Geometry check sheet. Reference: the model listing, model coordinates, mm. A direction names the side the tool comes from. Round coordinates to 2 decimals unless told otherwise and drop trailing zeros. Order: outer loops, then holes, each group sorted by start corner. A loop starts at its lowest first (then second) coordinate and runs counter-clockwise, first axis right, second up. Notation, with made-up numbers: M 78.5,-18 L 135.5,-18 A12 cw 135.5,4 Z; hole C -18.5,61 d5. An arc over 180 degrees is marked long. Return JSON: item names as keys, results as strings. Group by question number.
```python
from build123d import *

# Parameters (mm, degrees)
CUT_EXTRUDE1_DEPTH  = 12
SKETCH6_R           = 4.25
BOSS_EXTRUDE1_DEPTH = 5
SKETCH7_R           = 2.067
CUT_EXTRUDE2_DEPTH  = 40.361021372
SKETCH8_R           = 2.5
BOSS_EXTRUDE2_DEPTH = 18
CUT_EXTRUDE3_DEPTH  = 2
TAP1_D              = 4.134
TAP1_DEPTH          = 5.3


with BuildPart() as part:
    # Sketch1 → Revolve1 (revolve)
    with BuildSketch(Plane.XY, mode=Mode.PRIVATE) as revolve1_sk:
        Polygon((-26.6, -14), (-9.3, -14), (-9.3, -15.25), (-21.3, -15.75), (-21.3, -23), (-23.1, -23), (-23.1, -25), (-26.6, -25), align=None)
    revolve(revolve1_sk.sketch.rotate(Axis((0, 0, 0), (-1, 0, 0)), 180), axis=Axis((0, 0, 0), (-1, 0, 0)))

    # Sketch2 → Cut-Extrude1 (cut)
    with BuildSketch(Plane(origin=(-9.3, 0, 0), x_dir=(0, 0, -1), z_dir=(1, 0, 0))):
        with BuildLine():
            Line((0.5, -13.99106858), (0.5, -15.742061491))
            ThreePointArc((0.5, -15.742061491), (0, -15.75), (-0.5, -15.742061491))
            Line((-0.5, -15.742061491), (-0.5, -13.99106858))
            ThreePointArc((-0.5, -13.99106858), (0, -14), (0.5, -13.99106858))
        make_face()
    extrude(amount=-CUT_EXTRUDE1_DEPTH, mode=Mode.SUBTRACT)

    # Sketch3 → Revolve2 (revolve)
    with BuildSketch(Plane.XY, mode=Mode.PRIVATE) as revolve2_sk:
        Polygon((-17.3, -15.583333333), (0, -14.8625), (0, -23), (-17.3, -23), align=None)
    revolve(revolve2_sk.sketch.rotate(Axis((0, 0, 0), (-1, 0, 0)), 358.161317169), axis=Axis((0, 0, 0), (-1, 0, 0)))

    # Sketch4 for Cut-Loft1 → Cut-Loft1 section 0
    with BuildSketch(Plane(origin=(0, 0, 0), x_dir=(0, 0, -1), z_dir=(1, 0, 0))):
        with BuildLine():
            Line((6.531671834, 22.05305564), (4.288541607, 14.230330886))
            # circular arc as an exact rational Bezier (weights 1, cos(half-angle), 1)
            Bezier((4.288541607, 14.230330886), (4.097031168, 14.288045671), (3.904036928, 14.340585829), weights=[1, 0.999909455, 1])
            Line((3.904036928, 14.340585829), (6.147167155, 22.163310582))
            Bezier((6.147167155, 22.163310582), (6.339898882, 22.109854934), (6.531671834, 22.05305564), weights=[1, 0.999962192, 1])
        make_face()
    # Sketch5 for Cut-Loft1 → Cut-Loft1 section 1
    with BuildSketch(Plane.ZY.offset(17.3)):
        with BuildLine():
            Line((-6.531671834, 22.05305564), (-4.48724736, 14.923300202))
            Bezier((-4.48724736, 14.923300202), (-4.295702598, 14.980895286), (-4.102742682, 15.033555144), weights=[1, 0.999917638, 1])
            Line((-4.102742682, 15.033555144), (-6.147167155, 22.163310582))
            Bezier((-6.147167155, 22.163310582), (-6.339898882, 22.109854934), (-6.531671834, 22.05305564), weights=[1, 0.999962192, 1])
        make_face()
    loft(mode=Mode.SUBTRACT)

    # Sketch6 → Boss-Extrude1 (add)
    with BuildSketch(Plane.ZY.offset(26.6)):
        with Locations(Location((0, 19.4, 0), (0, 0, 90))):
            Circle(SKETCH6_R)
        with Locations(Location((10.280433726, -16.452133065, 0), (0, 0, 90))):
            Circle(SKETCH6_R)
        with Locations(Location((0, -19.4, 0), (0, 0, 90))):
            Circle(SKETCH6_R)
        with Locations(Location((-10.280433726, 16.452133065, 0), (0, 0, 90))):
            Circle(SKETCH6_R)
        with Locations(Location((10.280433726, 16.452133065, 0), (0, 0, 90))):
            Circle(SKETCH6_R)
        with Locations(Location((-10.280433726, -16.452133065, 0), (0, 0, 90))):
            Circle(SKETCH6_R)
        with Locations(Location((-18.648476901, 5.347364703, 0), (0, 0, 90))):
            Circle(SKETCH6_R)
        with Locations(Location((18.648476901, -5.347364703, 0), (0, 0, 90))):
            Circle(SKETCH6_R)
        with Locations(Location((18.648476901, 5.347364703, 0), (0, 0, 90))):
            Circle(SKETCH6_R)
        with Locations(Location((-18.648476901, -5.347364703, 0), (0, 0, 90))):
            Circle(SKETCH6_R)
    extrude(amount=BOSS_EXTRUDE1_DEPTH)

    # Sketch7 → Cut-Extrude2 (cut, through all)
    with BuildSketch(Plane.ZY.offset(17.3)):
        with Locations(Location((0, 19.4, 0), (0, 0, 270))):
            Circle(SKETCH7_R)
        with Locations(Location((10.280433726, -16.452133065, 0), (0, 0, 270))):
            Circle(SKETCH7_R)
        with Locations(Location((0, -19.4, 0), (0, 0, 270))):
            Circle(SKETCH7_R)
        with Locations(Location((-10.280433726, 16.452133065, 0), (0, 0, 270))):
            Circle(SKETCH7_R)
        with Locations(Location((10.280433726, 16.452133065, 0), (0, 0, 270))):
            Circle(SKETCH7_R)
        with Locations(Location((-10.280433726, -16.452133065, 0), (0, 0, 270))):
            Circle(SKETCH7_R)
        with Locations(Location((-18.648476901, 5.347364703, 0), (0, 0, 270))):
            Circle(SKETCH7_R)
        with Locations(Location((18.648476901, -5.347364703, 0), (0, 0, 270))):
            Circle(SKETCH7_R)
        with Locations(Location((18.648476901, 5.347364703, 0), (0, 0, 270))):
            Circle(SKETCH7_R)
        with Locations(Location((-18.648476901, -5.347364703, 0), (0, 0, 270))):
            Circle(SKETCH7_R)
    extrude(amount=-CUT_EXTRUDE2_DEPTH, mode=Mode.SUBTRACT)

    # Sketch8 → Boss-Extrude2 (add)
    with BuildSketch(Plane.ZY.offset(26.6)):
        with Locations(Location((0, 19.4, 0), (0, 0, 270))):
            Circle(SKETCH8_R)
        with Locations(Location((10.280433726, -16.452133065, 0), (0, 0, 270))):
            Circle(SKETCH8_R)
        with Locations(Location((0, -19.4, 0), (0, 0, 270))):
            Circle(SKETCH8_R)
        with Locations(Location((-10.280433726, 16.452133065, 0), (0, 0, 270))):
            Circle(SKETCH8_R)
        with Locations(Location((10.280433726, 16.452133065, 0), (0, 0, 270))):
            Circle(SKETCH8_R)
        with Locations(Location((-10.280433726, -16.452133065, 0), (0, 0, 270))):
            Circle(SKETCH8_R)
        with Locations(Location((-18.648476901, 5.347364703, 0), (0, 0, 270))):
            Circle(SKETCH8_R)
        with Locations(Location((18.648476901, -5.347364703, 0), (0, 0, 270))):
            Circle(SKETCH8_R)
        with Locations(Location((18.648476901, 5.347364703, 0), (0, 0, 270))):
            Circle(SKETCH8_R)
        with Locations(Location((-18.648476901, -5.347364703, 0), (0, 0, 270))):
            Circle(SKETCH8_R)
    extrude(amount=-BOSS_EXTRUDE2_DEPTH)

    # Sketch9 → Cut-Extrude3 (cut)
    with BuildSketch(Plane.ZY.offset(31.6)):
        Polygon((0, 21.709401077), (-2, 20.554700538), (-2, 18.245299462), (0, 17.090598923), (2, 18.245299462), (2, 20.554700538), align=None)
        Polygon((10.280433726, -14.142731989), (8.280433726, -15.297432527), (8.280433726, -17.606833604), (10.280433726, -18.761534142), (12.280433726, -17.606833604), (12.280433726, -15.297432527), align=None)
        Polygon((0, -17.090598923), (-2, -18.245299462), (-2, -20.554700538), (0, -21.709401077), (2, -20.554700538), (2, -18.245299462), align=None)
        Polygon((-10.280433726, 18.761534142), (-12.280433726, 17.606833604), (-12.280433726, 15.297432527), (-10.280433726, 14.142731989), (-8.280433726, 15.297432527), (-8.280433726, 17.606833604), align=None)
        Polygon((10.280433726, 18.761534142), (8.280433726, 17.606833604), (8.280433726, 15.297432527), (10.280433726, 14.142731989), (12.280433726, 15.297432527), (12.280433726, 17.606833604), align=None)
        Polygon((-10.280433726, -14.142731989), (-12.280433726, -15.297432527), (-12.280433726, -17.606833604), (-10.280433726, -18.761534142), (-8.280433726, -17.606833604), (-8.280433726, -15.297432527), align=None)
        Polygon((-18.648476901, 7.65676578), (-20.648476901, 6.502065241), (-20.648476901, 4.192664164), (-18.648476901, 3.037963626), (-16.648476901, 4.192664164), (-16.648476901, 6.502065241), align=None)
        Polygon((18.648476901, -3.037963626), (16.648476901, -4.192664164), (16.648476901, -6.502065241), (18.648476901, -7.65676578), (20.648476901, -6.502065241), (20.648476901, -4.192664164), align=None)
        Polygon((18.648476901, 7.65676578), (16.648476901, 6.502065241), (16.648476901, 4.192664164), (18.648476901, 3.037963626), (20.648476901, 4.192664164), (20.648476901, 6.502065241), align=None)
        Polygon((-18.648476901, -3.037963626), (-20.648476901, -4.192664164), (-20.648476901, -6.502065241), (-18.648476901, -7.65676578), (-16.648476901, -6.502065241), (-16.648476901, -4.192664164), align=None)
    extrude(amount=-CUT_EXTRUDE3_DEPTH, mode=Mode.SUBTRACT)

    # Tap1
    with Locations(Plane.ZY.offset(26.6)):
        with Locations((15.493528895, 11.675211449), (-15.493528895, -11.675211449), (-15.493528895, 11.675211449), (15.493528895, -11.675211449)):
            Hole(TAP1_D / 2, depth=TAP1_DEPTH)


solid = part.part
```
Q1. Set-up check for faces 4 (the face through (-29.065, -5.901, -22.862)), 5 (the face through (-15, -15, 0.5)), 6 (the face through (-8.6, -16, -10)): record each of +Z, -Z, +X, -X, +Y, -Y from which the full face is reachable in a straight line by a thin tool's end or side.
Q2. Depth check by flat-ended pin: pin 1 Ø1.5 at (x, z) = (-23.5, 2.5) entering from -Y; pin 2 Ø2 at (y, z) = (-20, -0.5) entering from +X; pin 3 Ø2 at (x, y) = (-30.5, 5.5) entering from +Z. Enter the tip coordinate at first touch or a pass-through.
Q3. Section check B-B on y = 0. Record the cut outline in (x, z).
Q4. Release check for a two-part mould opening along X. For faces 1 (the face through (-30.61, -18.19, 11.27)), 2 (the face through (-19.328, 18.436, 8.759)), 3 (the face through (0, -1, 16)) record: +X half, -X half, draft (parallel to the pull), parting line (faces both ways), or undercut.
Q5. Material ranges on line 1 along Z through (x, y) = (-4.75, -19.4); line 2 along X through (y, z) = (13, -12); line 3 along Z through (x, y) = (-26.5, 3), recorded low to high.
Q6. Section check A-A on x = -27.5. Count the separate pieces of the cut face and the enclosed holes in it, plus the area to 3 significant figures.
Geometry check:
{
 "1": {"face 4": "-X", "face 5": "none", "face 6": "+X"},
 "2": {"pin 1": "stops at y = -24.94", "pin 2": "stops at x = -8.6", "pin 3": "stops at z = 22.9"},
 "3": {"outline": "M -26.6,-25 L -23.1,-25 L -23.1,-23 L -21.3,-23 L -21.3,-15.75 L -17.3,-15.58 L -17.3,-23 L 0,-23 L 0,-14.86 L -9.3,-15.25 L -9.3,-14 L -26.6,-14 Z; M -26.6,14 L -9.3,14 L -9.3,15.25 L 0,14.86 L 0,23 L -17.3,23 L -17.3,15.58 L -21.3,15.75 L -21.3,23 L -23.1,23 L -23.1,25 L -26.6,25 Z"},
 "4": {"face 1": "draft", "face 2": "undercut", "face 3": "+X half"},
 "5": {"line 1": "z = -12.35 to -2.07, 2.07 to 12.35", "line 2": "x = -31.6 to -21.3, -17.3 to 0", "line 3": "z = -24.82 to -13.67, 13.67 to 24.82"},
 "6": {"separate pieces": "10", "enclosed holes": "0", "area": "567 mm^2"}
}
